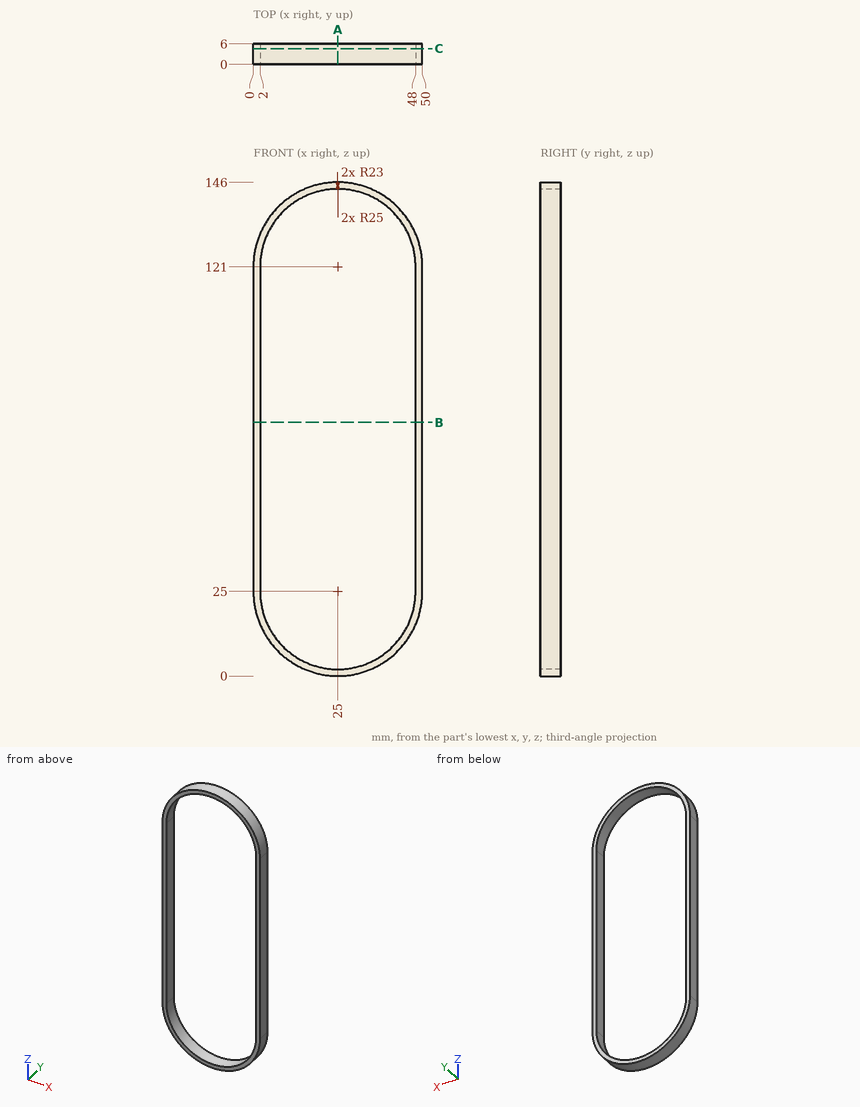
Design review of the part shown in the three views and the two pictorial views. Dimensions are in mm from the part's minimum x, y and z. Give positions to 0.01 mm unless a question says otherwise; leave off trailing zeros. Loops run counter-clockwise (first coordinate to the right, second up) from the corner with the lowest first, then second, coordinate; pieces in that order, holes last. Notation, with made-up numbers: (-7, 22.5) -> (15, 22.5) arc R6 cw to (15, 33.5) -> close; hole circle Ø11 at (60, 60.5). An arc over 180 degrees is marked (long way). Answer as a JSON object with one key per item and string values. Group by question number.
Q1. Wall thickness on line 1 along X through (y, z) = (0.35, 44); line 2 along Z through (x, y) = (37, 3.1); line 3 along X through (y, z) = (4.8, 17): over which ranges is each line inside the solid? List them lowest first.
Q2. Insertion check: pin 1 (1 mm diameter, centred on y = 3.5, z = 49.5, fed in from -X); pin 2 (1.5 mm diameter, centred on x = 34, y = 2.5, fed in from +Z). Each pin has a flat end and moves straight along its axis. Give the tip position at first contact, or say it passes through.
Q3. Take a section at B-B (z = 75). Write out the cut boundary in (x, y), plus the area to 3 significant figures.
Q4. Take a section at C-C (y = 4.65). Write out the cut boundary in (x, z).
Q5. Take a section at A-A (x = 25). Write out the cut boundary in (y, z), plus the area to 3 significant figures.
Answer below:
{
 "1": {"line 1": "x = 0 to 2, 48 to 50", "line 2": "z = 3.07 to 5.38, 140.62 to 142.93", "line 3": "x = 1.31 to 3.44, 46.56 to 48.69"},
 "2": {"pin 1": "stops at x = 0", "pin 2": "stops at z = 144.6"},
 "3": {"outline": "(0, 0) -> (2, 0) -> (2, 6) -> (0, 6) -> close; (48, 0) -> (50, 0) -> (50, 6) -> (48, 6) -> close", "area": "24.0 mm2"},
 "4": {"outline": "(0, 25) arc R25 ccw to (50, 25) -> (50, 121) arc R25 ccw to (0, 121) -> close; hole (2, 25) arc R23 ccw to (48, 25) -> (48, 121) arc R23 ccw to (2, 121) -> close"},
 "5": {"outline": "(0, 0) -> (6, 0) -> (6, 2) -> (0, 2) -> close; (0, 144) -> (6, 144) -> (6, 146) -> (0, 146) -> close", "area": "24.0 mm2"}
}
